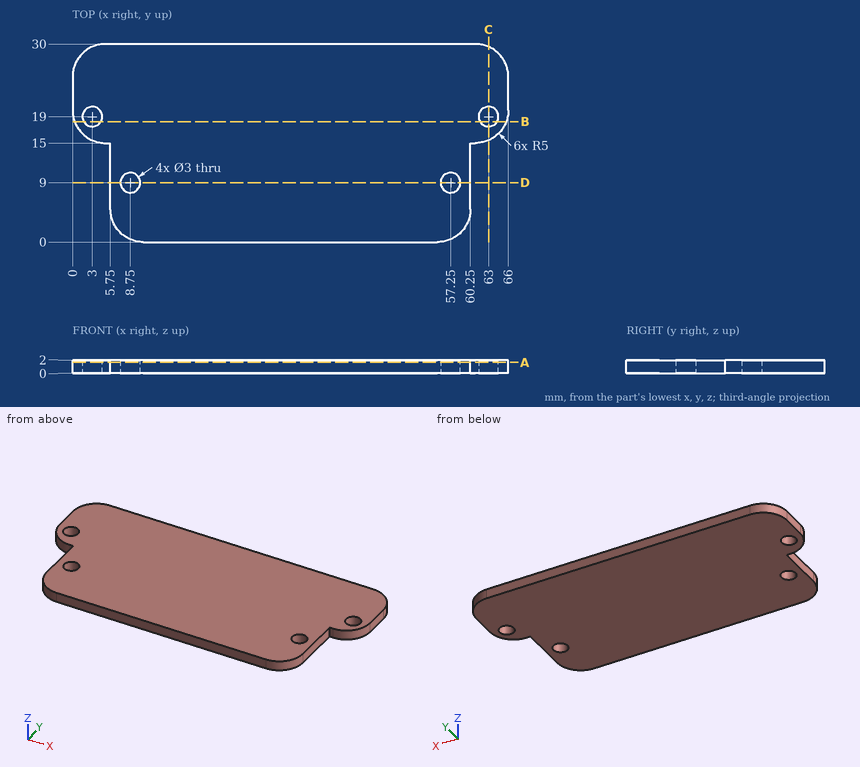
Print and shaded views of the part. All mm, measured from the part's lowest x, y and z. Give positions to 0.01 mm unless a question says otherwise; leave off trailing zeros. Write each loop counter-clockwise with the first axis right and the second up, starting at its lowest first coordinate (ties: lowest second). Pieces come first, ordered by that corner, then holes. Notation, with made-up numbers: (-25.75, -12) -> (14.25, -12) arc R20 cw to (14.25, 3) -> close; hole circle Ø7 at (87, 75.25). An arc over 180 degrees is marked (long way). Use CSV: the item, a comma, the result in double quotes. Start each with the question number.
1) Cut at B-B on y = 18.25. List the corners of the cut face in (x, z).
2) Drill centre lines: L1, parallel to X at y = 10, z = 1.8; L2, parallel to X at y = 12, z = 0.5; L3, parallel to X at y = 18.25, z = 1.75. Where is each one in solid material? Low to high.
3) Cut at C-C on x = 63. List the corners of the cut face in (y, z).
4) Pin check, flat tips, straight feed: P1, Ø4, axis at x = 3, y = 19, coming from the -Z side; P2, Ø2.5, axis at x = 63, y = 19, coming from the -Z side; P3, Ø1, axis at y = 10, z = 0, coming from the -X side; P4, Ø1, axis at y = 6, z = 0.5, coming from the +X side. Stop position of each tip, or through.
5) Cut at D-D on y = 9. List the corners of the cut face in (x, z).
6) Cut at A-A on z = 1.65. List the corners of the cut face in (x, y).
Final values:
1,outline,"(0.32, 0) -> (1.7, 0) -> (1.7, 2) -> (0.32, 2) -> close; (4.3, 0) -> (61.7, 0) -> (61.7, 2) -> (4.3, 2) -> close; (64.3, 0) -> (65.68, 0) -> (65.68, 2) -> (64.3, 2) -> close"
2,L1,"x = 5.75 to 7.63, 9.87 to 56.13, 58.37 to 60.25"
2,L2,"x = 5.75 to 60.25"
2,L3,"x = 0.32 to 1.7, 4.3 to 61.7, 64.3 to 65.68"
3,outline,"(15.42, 0) -> (17.5, 0) -> (17.5, 2) -> (15.42, 2) -> close; (20.5, 0) -> (29.58, 0) -> (29.58, 2) -> (20.5, 2) -> close"
4,P1,"stops at z = 0"
4,P2,"passes through"
4,P3,"stops at x = 5.75"
4,P4,"stops at x = 60.25"
5,outline,"(5.75, 0) -> (7.25, 0) -> (7.25, 2) -> (5.75, 2) -> close; (10.25, 0) -> (55.75, 0) -> (55.75, 2) -> (10.25, 2) -> close; (58.75, 0) -> (60.25, 0) -> (60.25, 2) -> (58.75, 2) -> close"
6,outline,"(0, 20) arc R5 ccw to (5, 15) -> (5.75, 15) -> (5.75, 5) arc R5 ccw to (10.75, 0) -> (55.25, 0) arc R5 ccw to (60.25, 5) -> (60.25, 15) -> (61, 15) arc R5 ccw to (66, 20) -> (66, 25) arc R5 ccw to (61, 30) -> (5, 30) arc R5 ccw to (0, 25) -> close; hole circle Ø3 at (3, 19); hole circle Ø3 at (8.75, 9); hole circle Ø3 at (57.25, 9); hole circle Ø3 at (63, 19)"
